Answer from the drawing. Dimensions are ordinates in mm from the lowest x, y and z of the part. A direction names the side the tool comes from. Coordinates: 2 decimals unless noted, no trailing zeros. Write each loop counter-clockwise with the first axis right and the second up, starting at its lowest first coordinate (ties: lowest second). Pieces come first, ordered by that corner, then holes.
(1) The part is cut by section C-C, the plane z = 3.25. Determine the outline of the cut face in (x, y).
(2) Straight lines are drawn through the part: line 1 along Y through (x, z) = (3.5, 9.75); line 2 along Z through (x, y) = (4.25, 2); line 3 along Z through (x, y) = (7, 6). For each, find the intervals that lie inside material, in ascending order.
(3) Given pin 1 (2 mm diameter, centred on y = 7.5, z = 3.5, fed in from +X); pin 2 (5 mm diameter, centred on y = 6, z = 10, fed in from +X); pin 3 (2 mm diameter, centred on x = 8, z = 12.5, fed in from +Y), each flat-ended and moving along its own axis, determine where each tip first touches the part or whether it passes through.
(4) The part is cut by section D-D, the plane y = 1.25. Determine the outline of the cut face in (x, z).
(5) Which of the six approach directions +Z, -Z, +X, -X, +Y, -Y give full straight-line access (tool end or side, diameter ignored) to the marked faces 1 and 2?
(6) The part is cut by section A-A, the plane y = 5. Determine the outline of the cut face in (x, z), and give its area (3 significant figures).
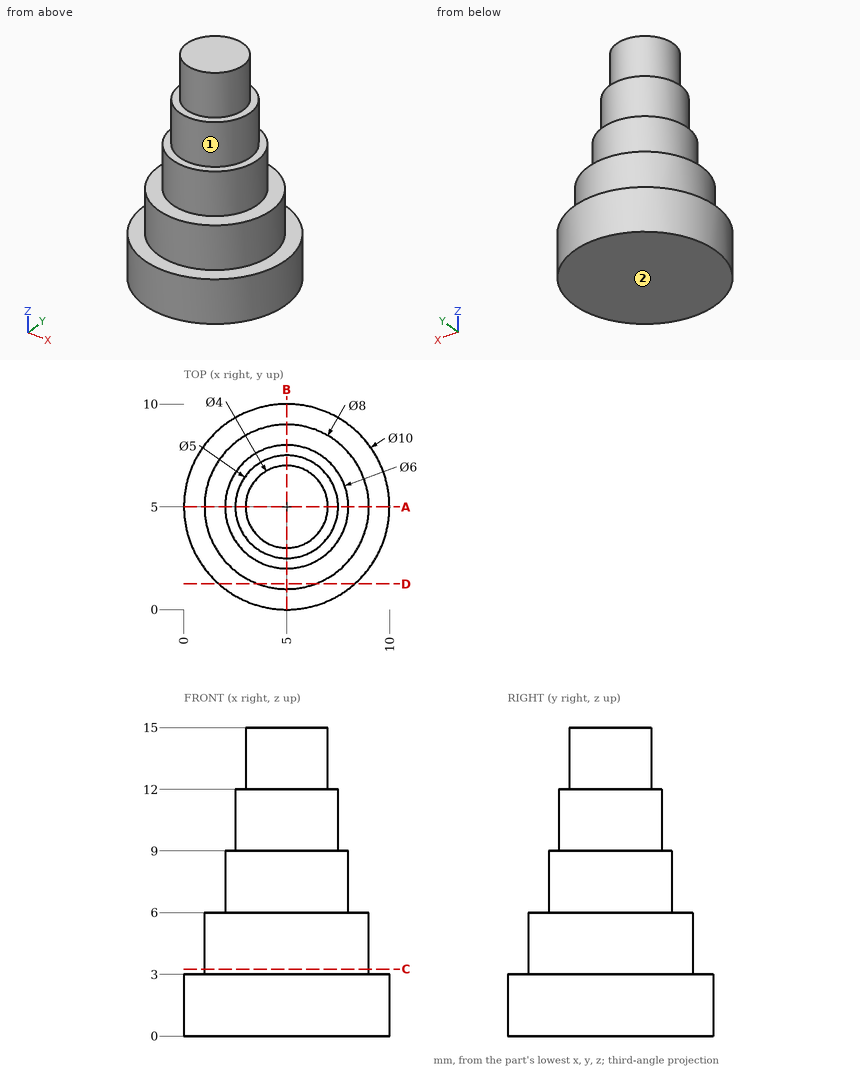
Computed:
1. outline: circle Ø8 at (5, 5)
2. line 1: y = 3 to 7
2. line 2: z = 0 to 6
2. line 3: z = 0 to 12
3. pin 1: stops at x = 9.73
3. pin 2: stops at x = 8
3. pin 3: stops at y = 6.3
4. outline: (1.69, 0) - (8.31, 0) - (8.31, 3) - (6.39, 3) - (6.39, 6) - (3.61, 6) - (3.61, 3) - (1.69, 3) - close
5. face 1: +Z
5. face 2: -Z, +X, -X, +Y, -Y
6. outline: (0, 0) - (10, 0) - (10, 3) - (9, 3) - (9, 6) - (8, 6) - (8, 9) - (7.5, 9) - (7.5, 12) - (7, 12) - (7, 15) - (3, 15) - (3, 12) - (2.5, 12) - (2.5, 9) - (2, 9) - (2, 6) - (1, 6) - (1, 3) - (0, 3) - close
6. area: 99.0 mm2
